Design review of the part shown in the three views and the two pictorial views. Dimensions are in mm from the part's minimum x, y and z. Coordinates: 2 decimals unless noted, no trailing zeros. Order: outer loops, then holes, each group sorted by start corner. A loop starts at its lowest first (then second) coordinate and runs counter-clockwise, first axis right, second up. Notation, with made-up numbers: (55, 31.25) - (106, 31.25) arc R21 ccw to (106, 49.25) - close; hole circle Ø10 at (-10, -20.75). An arc over 180 degrees is marked (long way). One line per item, written item: value. Start each with the question number.
(1) Consider section A-A on y = 80.2. Write out the cut boundary in (x, z).
(2) Clearance check with flat-ended pins moving along their axes: pin 1 (6.5 mm diameter, centred on x = 70, y = 5, fed in from -Z); pin 2 (4 mm diameter, centred on x = 5, y = 5, fed in from +Z). State where each tip first meets the part, or that it passes through.
(3) To check wall thickness, follow line 1 along X through (y, z) = (80.2, 8.3); line 2 along Y through (x, z) = (70, 1.8); line 3 along Y through (x, z) = (37.5, 2). State the ranges of each line that lie inside material, in increasing order.
(4) Consider section B-B on z = 3. Count the separate pieces of the cut face and the enclosed holes in it, then the cut area to 3 significant figures.
(5) Consider section C-C on y = 44.2. Write out the cut boundary in (x, z), then the cut area to 3 significant figures.
(6) Mouldability with a two-part tool opening along X and no side actions: class the marked faces 1, 2 and 3 as released by +X, released by -X, zero draft, split by the parting line, or undercut.
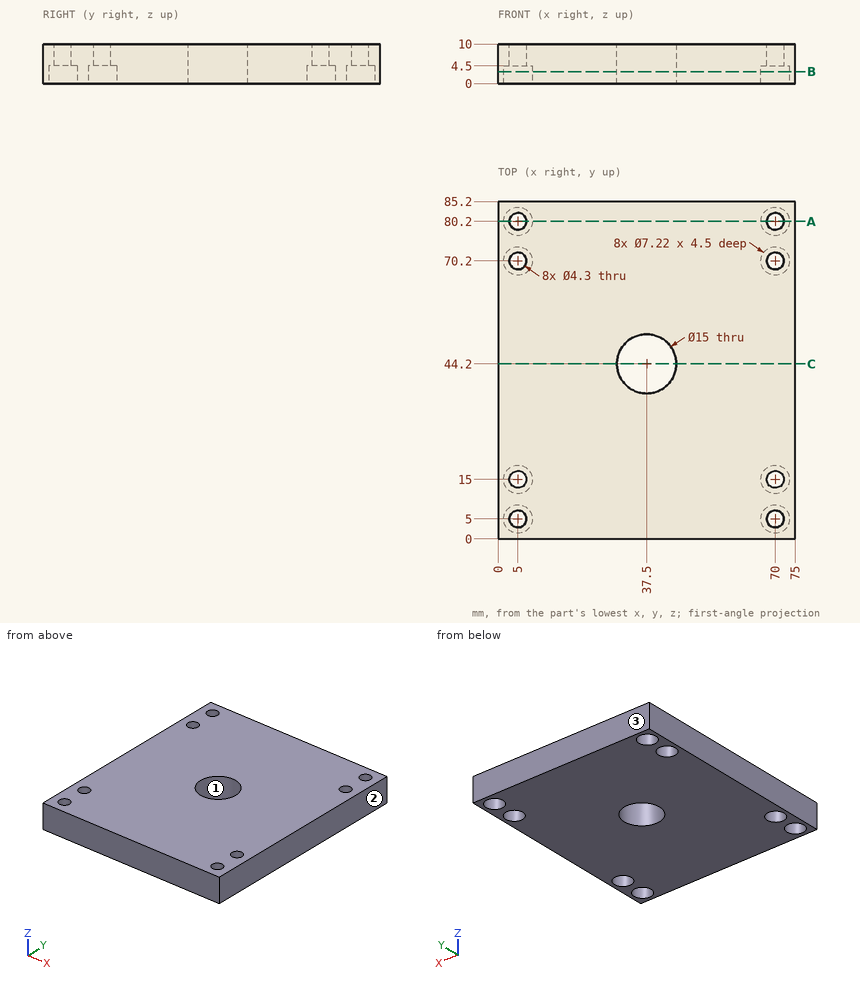
Geometry check:
1. outline: (0, 0) - (1.39, 0) - (1.39, 4.5) - (2.85, 4.5) - (2.85, 10) - (0, 10) - close; (7.15, 4.5) - (8.61, 4.5) - (8.61, 0) - (66.39, 0) - (66.39, 4.5) - (67.85, 4.5) - (67.85, 10) - (7.15, 10) - close; (72.15, 4.5) - (73.61, 4.5) - (73.61, 0) - (75, 0) - (75, 10) - (72.15, 10) - close
2. pin 1: stops at z = 4.5
2. pin 2: passes through
3. line 1: x = 0 to 2.85, 7.15 to 67.85, 72.15 to 75
3. line 2: y = 0 to 1.39, 8.61 to 11.39, 18.61 to 66.59, 73.81 to 76.59, 83.81 to 85.2
3. line 3: y = 0 to 36.7, 51.7 to 85.2
4. separate pieces: 1
4. enclosed holes: 9
4. area: 5,890 mm^2
5. outline: (0, 0) - (30, 0) - (30, 10) - (0, 10) - close; (45, 0) - (75, 0) - (75, 10) - (45, 10) - close
5. area: 600 mm^2
6. face 1: undercut
6. face 2: released by +X
6. face 3: zero draft
